Read the model definition and answer for the solid it produces. Units are mm, in the model's axes. Coordinates: 2 decimals unless noted, no trailing zeros. Write each loop counter-clockwise with the first axis right and the second up, starting at its lowest first coordinate (ties: lowest second). Pieces come first, ordered by that corner, then holes.
from build123d import *

# Parameters (mm, degrees)
ESQUISSE2_W             = 62
ESQUISSE2_H             = 44
ENL_V_MAT_EXTRU_1_DEPTH = 6.440596868
ESQUISSE3_W             = 6
ESQUISSE3_H             = 7
ESQUISSE3_W_2           = 7
ESQUISSE3_H_2           = 6
ENL_V_MAT_EXTRU_2_DEPTH = 3
ENL_V_MAT_EXTRU_3_DEPTH = 6.440596868
CHANFREIN1_SIZE         = 0.8


with BuildPart() as part:
    # Esquisse1 → Révolution1 (revolve)
    with BuildSketch(Plane.XY, mode=Mode.PRIVATE) as r_volution1_sk:
        with BuildLine():
            Line((37.6, 0), (37.6, 2))
            Line((37.6, 2), (34.9, 2))
            Line((34.9, 2), (34.9, 8.440596868))
            Line((34.9, 8.440596868), (48.6, 8.440596868))
            ThreePointArc((48.6, 8.440596868), (44.532598277, 2.35330001), (37.6, 0))
        make_face()
    revolve(r_volution1_sk.sketch.rotate(Axis((0, 0, 0), (0, 1, 0)), 90), axis=Axis((0, 0, 0), (0, 1, 0)))

    # Esquisse2 → Enlèv. mat.-Extru.1 (cut)
    with BuildSketch(Plane(origin=(0, 8.440596868, 0), x_dir=(1, 0, 0), z_dir=(0, 1, 0))):
        Rectangle(ESQUISSE2_W, ESQUISSE2_H)
    extrude(amount=-ENL_V_MAT_EXTRU_1_DEPTH, mode=Mode.SUBTRACT)

    # Esquisse3 → Enlèv. mat.-Extru.2 (cut)
    with BuildSketch(Plane(origin=(0, 8.440596868, 0), x_dir=(1, 0, 0), z_dir=(0, 1, 0))):
        with Locations((0, 42.1)):
            Rectangle(ESQUISSE3_W, ESQUISSE3_H)
        Polygon((8.891430026, 44.774378523), (14.686984983, 43.221464252), (12.875251668, 36.459983468), (7.07969671, 38.012897739), align=None)
        Polygon((20.163982836, 40.899160851), (25.360135259, 37.899160851), (21.860135259, 31.836983025), (16.663982836, 34.836983025), align=None)
        Polygon((30.049452587, 34.238436665), (34.292093274, 29.995795978), (29.342345806, 25.04604851), (25.099705119, 29.288689197), align=None)
        Polygon((37.874160851, 25.246123311), (40.874160851, 20.049970888), (34.811983025, 16.549970888), (31.811983025, 21.746123311), align=None)
        Polygon((43.104866691, 14.535032083), (44.657780961, 8.739477125), (37.896300177, 6.927743809), (36.343385907, 12.723298767), align=None)
        with Locations((41.885106147, -0.164893853)):
            Rectangle(ESQUISSE3_W_2, ESQUISSE3_H_2)
        Polygon((44.55948467, -9.056323878), (43.006570399, -14.851878836), (36.245089615, -13.04014552), (37.798003886, -7.244590563), align=None)
        Polygon((40.684266998, -20.328876689), (37.684266998, -25.525029112), (31.622089172, -22.025029112), (34.622089172, -16.828876689), align=None)
        Polygon((34.023542812, -30.21434644), (29.780902125, -34.456987127), (24.831154657, -29.507239659), (29.073795344, -25.264598972), align=None)
        Polygon((25.031229458, -38.039054704), (19.835077035, -41.039054704), (16.335077035, -34.976876877), (21.531229458, -31.976876877), align=None)
        Polygon((14.32013823, -43.269760543), (8.524583272, -44.822674814), (6.712849956, -38.06119403), (12.508404914, -36.508279759), align=None)
        with Locations((-0.379787706, -42.05)):
            Rectangle(ESQUISSE3_W, ESQUISSE3_H)
        Polygon((-9.271217731, -44.724378523), (-15.066772689, -43.171464252), (-13.255039373, -36.409983468), (-7.459484415, -37.962897739), align=None)
        Polygon((-20.543770542, -40.849160851), (-25.739922965, -37.849160851), (-22.239922965, -31.786983025), (-17.043770542, -34.786983025), align=None)
        Polygon((-30.429240293, -34.188436665), (-34.67188098, -29.945795978), (-29.722133512, -24.99604851), (-25.479492825, -29.238689197), align=None)
        Polygon((-38.253948557, -25.196123311), (-41.253948557, -19.999970888), (-35.19177073, -16.499970888), (-32.19177073, -21.696123311), align=None)
        Polygon((-43.484654396, -14.485032083), (-45.037568667, -8.689477125), (-38.276087883, -6.877743809), (-36.723173612, -12.673298767), align=None)
        with Locations((-42.264893853, 0.214893853)):
            Rectangle(ESQUISSE3_W_2, ESQUISSE3_H_2)
        Polygon((-44.939272376, 9.106323878), (-43.386358105, 14.901878836), (-36.624877321, 13.09014552), (-38.177791592, 7.294590563), align=None)
        Polygon((-41.064054704, 20.378876689), (-38.064054704, 25.575029112), (-32.001876877, 22.075029112), (-35.001876877, 16.878876689), align=None)
        Polygon((-34.403330518, 30.26434644), (-30.160689831, 34.506987127), (-25.210942362, 29.557239659), (-29.45358305, 25.314598972), align=None)
        Polygon((-25.411017164, 38.089054704), (-20.214864741, 41.089054704), (-16.714864741, 35.026876877), (-21.911017164, 32.026876877), align=None)
        Polygon((-14.699925936, 43.319760543), (-8.904370978, 44.872674814), (-7.092637662, 38.11119403), (-12.88819262, 36.558279759), align=None)
    extrude(amount=-ENL_V_MAT_EXTRU_2_DEPTH, mode=Mode.SUBTRACT)

    # Esquisse4 → Enlèv. mat.-Extru.3 (cut)
    with BuildSketch(Plane(origin=(0, 8.440596868, 0), x_dir=(1, 0, 0), z_dir=(0, 1, 0))):
        with BuildLine():
            Line((-1.5, 36.567750143), (-1.5, 34.867750143))
            Line((-1.5, 34.867750143), (1.5, 34.867750143))
            Line((1.5, 34.867750143), (1.5, 36.567750143))
            ThreePointArc((1.5, 36.567750143), (0, 38.067750143), (-1.5, 36.567750143))
        make_face()
    extrude(amount=-ENL_V_MAT_EXTRU_3_DEPTH, mode=Mode.SUBTRACT)

    # Chanfrein1
    chanfrein1_edges = [part.edges().sort_by_distance(p)[0] for p in [
        (34.9, 8.440596868, 0),
        (0, 8.440596868, 34.9),
        (-34.9, 8.440596868, 0),
        (-15.677347117, 8.440596868, -31.180615571),
        (15.677347117, 8.440596868, -31.180615571),
    ]]
    chamfer(chanfrein1_edges, length=CHANFREIN1_SIZE)


solid = part.part
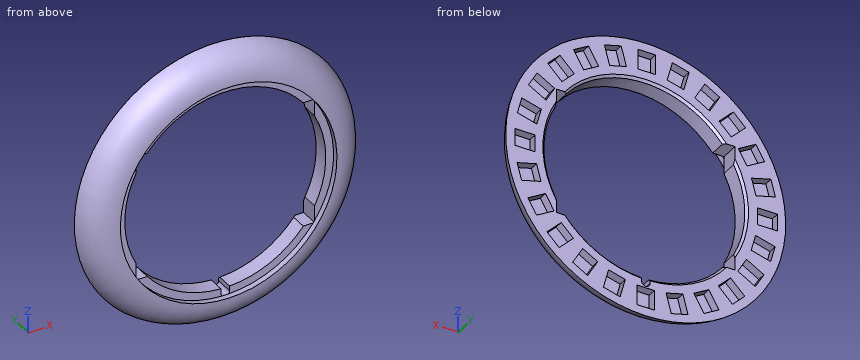
Item 1: Find the intervals of material crossed by probe 1 along Z at (x, y) = (22.5, 7.75); probe 2 along Z at (x, y) = (20, 8.25); probe 3 along X at (y, z) = (1.5, 0), in increasing order.
Item 2: The part is cut by section A-A (x = 0). Give the vertices of the cut face in (y, z), and give its area (3 significant figures).
Item 3: The part is cut by section B-B (z = 0). Give the vertices of the cut face in (x, y).
Item 4: Given pin 1 (9.5 mm diameter, centred on x = -19.5, z = -35.5, fed in from +Y); pin 2 (1.5 mm diameter, centred on y = 7, z = 0.5, fed in from -X); pin 3 (2.5 mm diameter, centred on x = 10, z = -40, fed in from +Y); pin 4 (4.5 mm diameter, centred on x = -21.5, z = -26, fed in from -Y), each flat-ended and moving along its own axis, determine where each tip first touches the part or whether it passes through.
Item 5: The part is cut by section C-C (y = 3.25). Give the vertices of the cut face in (x, z).
Answer:
1. probe 1: z = -42.84 to -39.55, -32.95 to -26.82, 26.82 to 33.65, 39.5 to 42.84
1. probe 2: z = -44.24 to -40.62, -32.91 to -29.34, 29.34 to 32.86, 40.94 to 44.24
1. probe 3: x = -43.25 to -37.6, 37.6 to 43.25
2. outline: (0, -37.6) arc R11.39 ccw to (8.44, -48.6) - (8.44, -45.6) - (5.44, -45.6) - (5.44, -38.6) - (8.44, -38.6) - (8.44, -38.07) - (2, -38.07) - (2, -37.6) - close; (0, 37.6) - (2, 37.6) - (2, 34.9) - (7.64, 34.9) - (8.44, 35.7) - (8.44, 38.55) - (5.44, 38.55) - (5.44, 45.55) - (8.44, 45.55) - (8.44, 48.6) arc R11.39 ccw to start
2. area: 109 mm2
3. outline: (-48.6, 8.44) arc R11.39 ccw to (-37.6, 0) - (-37.6, 2) - (-34.9, 2) - (-34.9, 7.64) - (-35.7, 8.44) - (-38.76, 8.44) - (-38.76, 5.44) - (-45.76, 5.44) - (-45.76, 8.44) - close; (34.9, 2) - (37.6, 2) - (37.6, 0) arc R11.39 ccw to (48.6, 8.44) - (45.39, 8.44) - (45.39, 5.44) - (38.39, 5.44) - (38.39, 8.44) - (35.7, 8.44) - (34.9, 7.64) - close
4. pin 1: stops at y = 8.44
4. pin 2: stops at x = -48.39
4. pin 3: stops at y = 5.44
4. pin 4: stops at y = 2
5. outline: circle Ø91.13 at (0, 0); hole (-31, -22) - (-27.09, -22) arc R34.9 ccw to (-1.5, -34.87) - (-1.5, -36.57) arc R1.5 ccw to (1.5, -36.57) - (1.5, -34.87) arc R34.9 ccw to (27.09, -22) - (31, -22) - (31, -16.03) arc R34.9 ccw to (31, 16.03) - (31, 22) - (27.09, 22) arc R34.9 ccw to (-27.09, 22) - (-31, 22) - (-31, 16.03) arc R34.9 ccw to (-31, -16.03) - close
